Here's the drawing with two shaded views (mm, measured from the low corner). I have some questions. Coordinates: 2 decimals unless noted, no trailing zeros. Order: outer loops, then holes, each group sorted by start corner. A loop starts at its lowest first (then second) coordinate and runs counter-clockwise, first axis right, second up. Notation, with made-up numbers: (17.25, 33.25) -> (75.25, 33.25) arc R19 ccw to (75.25, 53.25) -> close; hole circle Ø3 at (33.25, 66.5). An arc over 180 degrees is marked (long way). Answer in a Markdown table with one row per item. Add a question column.
1. Imagine slicing it at D-D on x = 3.5. Write out the boundary of the cut face in (y, z), plus the area to 3 significant figures.
2. Imagine slicing it at A-A on z = 38.5. Write out the boundary of the cut face in (x, y).
3. Will this pin go through, and if not, where does the flat tip stop? pin 1 (1 mm diameter, centred on x = 10.5, y = 2, fed in from +Z).
4. Imagine slicing it at B-B on y = 0.8. Write out the boundary of the cut face in (x, z), plus the area to 3 significant figures.
5. Imagine slicing it at C-C on x = 10. Write out the boundary of the cut face in (y, z), plus the area to 3 significant figures.
6. If I drill on line 1 along X through (y, z) = (2.8, 30); line 2 along X through (y, z) = (0.25, 3); line 3 along Z through (x, y) = (6.75, 1.35), over which ranges is the centre line in solid material (lowest first)? Write a range as [from, to].
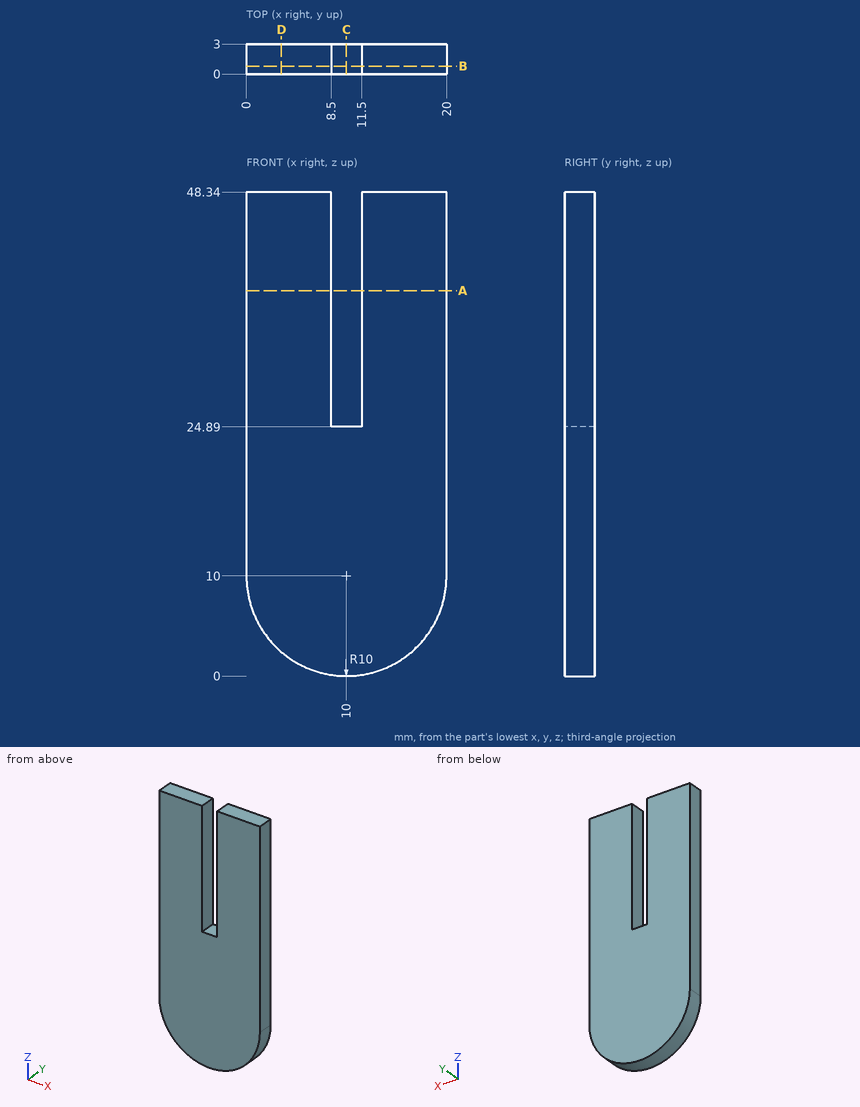
Answers follow:
| question | item | result |
|---|---|---|
| 1 | outline | (0, 2.4) -> (3, 2.4) -> (3, 48.34) -> (0, 48.34) -> close |
| 1 | area | 138 mm² |
| 2 | outline | (0, 0) -> (8.5, 0) -> (8.5, 3) -> (0, 3) -> close; (11.5, 0) -> (20, 0) -> (20, 3) -> (11.5, 3) -> close |
| 3 | pin 1 | stops at z = 24.89 |
| 4 | outline | (0, 10) arc R10 ccw to (20, 10) -> (20, 48.34) -> (11.5, 48.34) -> (11.5, 24.89) -> (8.5, 24.89) -> (8.5, 48.34) -> (0, 48.34) -> close |
| 4 | area | 854 mm² |
| 5 | outline | (0, 0) -> (3, 0) -> (3, 24.89) -> (0, 24.89) -> close |
| 5 | area | 74.7 mm² |
| 6 | line 1 | x = [0, 8.5], [11.5, 20] |
| 6 | line 2 | x = [2.86, 17.14] |
| 6 | line 3 | z = [0.54, 48.34] |
